from build123d import *

# Parameters (mm, degrees)
F0_R     = 1.75
F1_DEPTH = 6
F3_DEPTH = 5
F4_W     = 1.5
F4_H     = 5
F5_DEPTH = 5


with BuildPart() as f1:
    # F0 (on Front) → F1 (new body)
    with BuildSketch(Plane.XZ):
        with BuildLine():
            Line((23.236779, 1.51637), (13.06236, 10.26637))
            ThreePointArc((13.06236, 10.26637), (12.453716, 10.625199), (11.758281, 10.75))
            Line((11.758281, 10.75), (0, 10.75))
            Line((0, 10.75), (-11.758281, 10.75))
            ThreePointArc((-11.758281, 10.75), (-12.453716, 10.625199), (-13.06236, 10.26637))
            Line((-13.06236, 10.26637), (-23.236779, 1.51637))
            ThreePointArc((-23.236779, 1.51637), (-23.9327, 0), (-23.236779, -1.51637))
            Line((-23.236779, -1.51637), (-13.06236, -10.26637))
            ThreePointArc((-13.06236, -10.26637), (-12.453716, -10.625199), (-11.758281, -10.75))
            Line((-11.758281, -10.75), (0, -10.75))
            Line((0, -10.75), (11.758281, -10.75))
            ThreePointArc((11.758281, -10.75), (12.453716, -10.625199), (13.06236, -10.26637))
            Line((13.06236, -10.26637), (23.236779, -1.51637))
            ThreePointArc((23.236779, -1.51637), (23.9327, 0), (23.236779, 1.51637))
        make_face()
        with Locations((-20, 0)):
            Circle(F0_R, mode=Mode.SUBTRACT)
        with Locations((20, 0)):
            Circle(F0_R, mode=Mode.SUBTRACT)
    extrude(amount=F1_DEPTH)

    # F2 (on face) → F3 (cut)
    with BuildSketch(Plane.XZ.offset(6)):
        with BuildLine():
            Line((-13.5, 5.933183), (-13.5, -6.5))
            ThreePointArc((-13.5, -6.5), (-12.62132, -8.62132), (-10.5, -9.5))
            Line((-10.5, -9.5), (10.5, -9.5))
            ThreePointArc((10.5, -9.5), (12.62132, -8.62132), (13.5, -6.5))
            Line((13.5, -6.5), (13.5, 5.933183))
            Line((13.5, 5.933183), (9.352538, 9.5))
            Line((9.352538, 9.5), (-9.352538, 9.5))
            Line((-9.352538, 9.5), (-13.5, 5.933183))
        make_face()
    extrude(amount=-F3_DEPTH, mode=Mode.SUBTRACT)

    # F4 (on face) → F5 (join)
    with BuildSketch(Plane.XZ.offset(1)):
        with Locations((0, -4.298508)):
            Rectangle(F4_W, F4_H)
        with Locations((-8, 0)):
            Rectangle(F4_W, F4_H)
        with Locations((8, 0)):
            Rectangle(F4_W, F4_H)
    extrude(amount=F5_DEPTH)


solid = f1.part
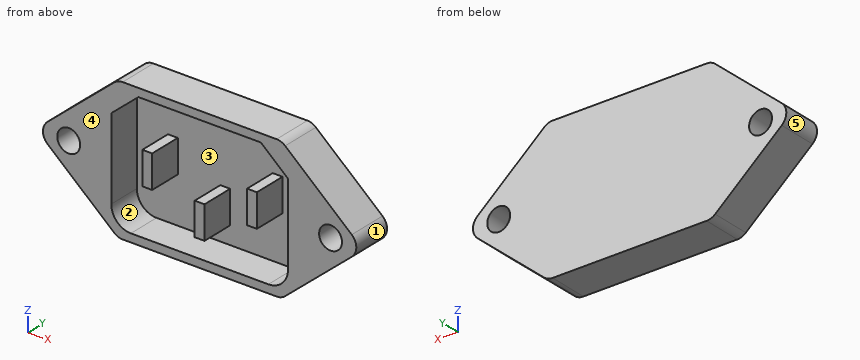
Part model, mm, in its own coordinate system. Face numbers are marked on the shaded views. A direction names the side the tool comes from. Give positions to 0.01 mm unless a question says otherwise; leave off trailing zeros. Order: outer loops, then holes, each group sorted by start corner. A loop starts at its lowest first (then second) coordinate and runs counter-clockwise, first axis right, second up. Notation, with made-up numbers: (82, 76.25) - (90, 76.25) arc R18 ccw to (90, 89.25) - close; hole circle Ø10 at (0, 23.25). An arc over 180 degrees is marked (long way). Use a Markdown table: item, result.
1) Flat gauge pins, fed straight in: P1, Ø5.5, axis at x = -20, z = 0, coming from the +Y side; P2, Ø3, axis at y = -2.5, z = 5, coming from the +X side; P3, Ø1, axis at y = -5, z = -6, coming from the +X side; P4, Ø2.5, axis at y = -4.5, z = -2, coming from the +X side. Where does each tip first touch, or does it go through?
Checked values:
| item | result |
|---|---|
| P1 | y = 0 |
| P2 | x = 20.93 |
| P3 | x = 18.6 |
| P4 | x = 23.79 |
2) Probe L1, parallel to Z at x = 8.5, y = -3.2; L2, parallel to X at y = -3.2, z = 1; L3, parallel to X at y = -4.8, z = 8.5. List the from-to ranges inside material, lowest first. Write a range as from..to.
Checked values:
| item | result |
|---|---|
| L1 | -10.75..-9.5, -2.5..2.5, 9.5..10.75 |
| L2 | -23.66..-21.44, -18.56..-13.5, -8.75..-7.25, 7.25..8.75, 13.5..18.56, 21.44..23.66 |
| L3 | -15.12..-10.52, 10.52..15.12 |
3) Saw through at B-B on x = 20. List the corners of the cut face in (y, z).
Checked values:
| item | result |
|---|---|
| outline | (-6, -4.3) - (0, -4.3) - (0, -1.75) - (-6, -1.75) - close; (-6, 1.75) - (0, 1.75) - (0, 4.3) - (-6, 4.3) - close |
4) Saw through at C-C on z = 0. List the corners of the cut face in (x, y).
Checked values:
| item | result |
|---|---|
| outline | (-23.93, -6) - (-21.75, -6) - (-21.75, 0) - (-23.93, 0) - close; (-18.25, -6) - (-13.5, -6) - (-13.5, -1) - (-8.75, -1) - (-8.75, -6) - (-7.25, -6) - (-7.25, -1) - (7.25, -1) - (7.25, -6) - (8.75, -6) - (8.75, -1) - (13.5, -1) - (13.5, -6) - (18.25, -6) - (18.25, 0) - (-18.25, 0) - close; (21.75, -6) - (23.93, -6) - (23.93, 0) - (21.75, 0) - close |
5) Saw through at D-D on x = 0. List the corners of the cut face in (y, z).
Checked values:
| item | result |
|---|---|
| outline | (-6, -10.75) - (0, -10.75) - (0, 10.75) - (-6, 10.75) - (-6, 9.5) - (-1, 9.5) - (-1, -1.8) - (-6, -1.8) - (-6, -6.8) - (-1, -6.8) - (-1, -9.5) - (-6, -9.5) - close |
6) Saw through at A-A on y = -3.85. Count the separate pieces of the cut face and the enclosed holes in it, plus the area to 3 significant figures.
Checked values:
| item | result |
|---|---|
| separate pieces | 4 |
| enclosed holes | 3 |
| area | 312 mm² |
7) 3-axis set-ups, long thin cutter, end or side, ignore diameter. For the marked faces 1 and 2: which of +Z, -Z, +X, -X, +Y, -Y reach the whole face in a straight line?
Checked values:
| item | result |
|---|---|
| face 1 | +X, +Y, -Y |
| face 2 | -Y |
8) Two-plate mould, pull along X, no slides. Class the marked faces 3, 4 and 5: +X half, -X half, draft (parallel to the pull), parting line (faces both ways), or undercut.
Checked values:
| item | result |
|---|---|
| face 3 | undercut |
| face 4 | draft |
| face 5 | -X half |
